Can you work these out from the model? Positions are in its coordinate system, mm. A direction names the side the tool comes from. Coordinates: 2 decimals unless noted, no trailing zeros. Order: outer loops, then holes, each group sorted by start corner. A loop starts at its lowest first (then second) coordinate and runs counter-clockwise, first axis right, second up. Notation, with made-up numbers: M 64.5,-38 L 72.5,-38 A25 cw 72.5,-22 Z; hole C 77.5,72.25 d2. An arc over 180 degrees is marked long. Answer as a JSON object with one key per item and string values.
from build123d import *

# Parameters (mm, degrees)
SKETCH1_R                           = 97.5
PLATE_DEPTH                         = 2
SKETCH2_W                           = 38
SKETCH2_H                           = 38
FIN_CLEARANCES_DEPTH                = 2
SKETCH3_W                           = 17.168411885
SKETCH3_H                           = 21
SERVO_CLEARANCE_DEPTH               = 2
SKETCH4_W                           = 4
SKETCH4_H                           = 21
SERVO_LIP_BOTTOM_DEPTH              = 8
SKETCH5_W                           = 10.5
SKETCH5_H                           = 5
SERVO_LIP_TOP_EXTRUSION_DEPTH       = 52
SKETCH6_W                           = 10.5
SKETCH6_H                           = 11.9
SERVO_LIP_TOP_DEPTH                 = 20.75
SKETCH7_W                           = 35
SKETCH7_H                           = 21
SERVO_CLEARANCE_FOR_INSERTION_DEPTH = 2
F_4_SERVO_LIP_EXTRUSIONS_COUNT      = 4
SKETCH8_W                           = 10.5
SKETCH8_H                           = 11.9
BOSS_EXTRUDE6_DEPTH                 = 20.75
SKETCH9_W                           = 10.5
SKETCH9_H                           = 11.9
BOSS_EXTRUDE7_DEPTH                 = 20.75
SKETCH10_W                          = 10.5
SKETCH10_H                          = 11.9
BOSS_EXTRUDE8_DEPTH                 = 20.75
SKETCH11_W                          = 5
SKETCH11_H                          = 55
EBOX_LID_SUPPORT_DEPTH              = 50
CUT_EXTRUDE4_DEPTH                  = 2
CLIP_CLEARANCES_COUNT               = 4
SKETCH13_W                          = 6
SKETCH13_H                          = 89.5
EBOX_BOTTOM_SUPPORT_DEPTH           = 20
SKETCH14_W                          = 22
SKETCH14_H                          = 5
SKETCH14_W_2                        = 3
SKETCH14_H_2                        = 8
CUT_EXTRUDE5_DEPTH                  = 10
CIRPATTERN1_COUNT                   = 4


with BuildPart() as part:
    # Sketch1 → Plate (new body)
    with BuildSketch(Plane(origin=(0, 0, 0), x_dir=(1, 0, 0), z_dir=(0, 1, 0))):
        with Locations(Location((0, 0, 0), (0, 0, 270))):
            Circle(SKETCH1_R)
    extrude(amount=PLATE_DEPTH)

    # Sketch2 → Fin Clearances (cut)
    with BuildSketch(Plane(origin=(0, 2, 0), x_dir=(1, 0, 0), z_dir=(0, 1, 0))):
        with Locations((69, 0)):
            Rectangle(SKETCH2_W, SKETCH2_H)
        with Locations((0, 69)):
            Rectangle(SKETCH2_W, SKETCH2_H)
        with Locations((0, -69)):
            Rectangle(SKETCH2_W, SKETCH2_H)
        with Locations((-69, 0)):
            Rectangle(SKETCH2_W, SKETCH2_H)
    extrude(amount=-FIN_CLEARANCES_DEPTH, mode=Mode.SUBTRACT)

    # Sketch3 → Servo Clearance (cut)
    with BuildSketch(Plane.XZ):
        with Locations((-27.584205943, -55.25)):
            Rectangle(SKETCH3_W, SKETCH3_H)
    servo_clearance = extrude(amount=-SERVO_CLEARANCE_DEPTH, mode=Mode.SUBTRACT)

    # Sketch4 → Servo Lip - Bottom (add)
    with BuildSketch(Plane.XZ):
        with Locations((-38.168411885, -55.25)):
            Rectangle(SKETCH4_W, SKETCH4_H)
    servo_lip_bottom = extrude(amount=SERVO_LIP_BOTTOM_DEPTH)

    # Sketch5 → Servo Lip - Top Extrusion (add)
    with BuildSketch(Plane(origin=(0, 2, 0), x_dir=(1, 0, 0), z_dir=(0, 1, 0))):
        with Locations((-41.418411885, 68.25)):
            Rectangle(SKETCH5_W, SKETCH5_H)
    servo_lip_top_extrusion = extrude(amount=SERVO_LIP_TOP_EXTRUSION_DEPTH)

    # Sketch6 → Servo Lip - Top (add)
    with BuildSketch(Plane.XY.offset(-65.75)):
        with Locations((-41.418411885, 48.05)):
            Rectangle(SKETCH6_W, SKETCH6_H)
    extrude(amount=SERVO_LIP_TOP_DEPTH)

    # Sketch7 → Servo Clearance for Insertion (cut)
    with BuildSketch(Plane.XZ):
        with Locations((-18.668411885, -55.25)):
            Rectangle(SKETCH7_W, SKETCH7_H)
    servo_clearance_for_insertion = extrude(amount=-SERVO_CLEARANCE_FOR_INSERTION_DEPTH, mode=Mode.SUBTRACT)

    # 4 Servo Lip Extrusions: Servo Clearance, Servo Lip - Bottom, Servo Lip - Top Extrusion, Servo Clearance for Insertion ×4 about axis
    f_4_servo_lip_extrusions_axis = Axis((0, 0, 0), (0, 1, 0))
    add([servo_clearance.rotate(f_4_servo_lip_extrusions_axis, i * 360 / F_4_SERVO_LIP_EXTRUSIONS_COUNT) for i in range(1, F_4_SERVO_LIP_EXTRUSIONS_COUNT)], mode=Mode.SUBTRACT)
    add([servo_lip_bottom.rotate(f_4_servo_lip_extrusions_axis, i * 360 / F_4_SERVO_LIP_EXTRUSIONS_COUNT) for i in range(1, F_4_SERVO_LIP_EXTRUSIONS_COUNT)])
    add([servo_lip_top_extrusion.rotate(f_4_servo_lip_extrusions_axis, i * 360 / F_4_SERVO_LIP_EXTRUSIONS_COUNT) for i in range(1, F_4_SERVO_LIP_EXTRUSIONS_COUNT)])
    add([servo_clearance_for_insertion.rotate(f_4_servo_lip_extrusions_axis, i * 360 / F_4_SERVO_LIP_EXTRUSIONS_COUNT) for i in range(1, F_4_SERVO_LIP_EXTRUSIONS_COUNT)], mode=Mode.SUBTRACT)

    # Sketch8 → Boss-Extrude6 (add)
    with BuildSketch(Plane(origin=(-65.75, 0, 0), x_dir=(0, 0, -1), z_dir=(1, 0, 0))):
        with Locations((-41.418411885, 48.05)):
            Rectangle(SKETCH8_W, SKETCH8_H)
    extrude(amount=BOSS_EXTRUDE6_DEPTH)

    # Sketch9 → Boss-Extrude7 (add)
    with BuildSketch(Plane(origin=(0, 0, 65.75), x_dir=(-1, 0, 0), z_dir=(0, 0, -1))):
        with Locations((-41.418411885, 48.05)):
            Rectangle(SKETCH9_W, SKETCH9_H)
    extrude(amount=BOSS_EXTRUDE7_DEPTH)

    # Sketch10 → Boss-Extrude8 (add)
    with BuildSketch(Plane.ZY.offset(-65.75)):
        with Locations((-41.418411885, 48.05)):
            Rectangle(SKETCH10_W, SKETCH10_H)
    extrude(amount=BOSS_EXTRUDE8_DEPTH)

    # Sketch11 → EBox Lid Support (add)
    with BuildSketch(Plane(origin=(0, 2, 0), x_dir=(1, 0, 0), z_dir=(0, 1, 0))):
        with Locations((-30.25, -1.627343475)):
            Rectangle(SKETCH11_W, SKETCH11_H)
    extrude(amount=EBOX_LID_SUPPORT_DEPTH)

    # Sketch12 → Cut-Extrude4 (cut)
    with BuildSketch(Plane.XZ):
        Polygon((-71.064231509, 63.993163697), (-63.993163697, 71.064231509), (-65.40737726, 72.478445072), (-72.478445072, 65.40737726), align=None)
    cut_extrude4 = extrude(amount=-CUT_EXTRUDE4_DEPTH, mode=Mode.SUBTRACT)

    # Clip Clearances: Cut-Extrude4 ×4 about axis
    clip_clearances_axis = Axis((0, 0, 0), (0, 1, 0))
    for i in range(1, CLIP_CLEARANCES_COUNT):
        add(cut_extrude4.rotate(clip_clearances_axis, i * 360 / CLIP_CLEARANCES_COUNT), mode=Mode.SUBTRACT)

    # Sketch13 → EBox Bottom Support (add)
    with BuildSketch(Plane(origin=(0, 2, 0), x_dir=(1, 0, 0), z_dir=(0, 1, 0))):
        with Locations((31, 0)):
            Rectangle(SKETCH13_W, SKETCH13_H)
    extrude(amount=EBOX_BOTTOM_SUPPORT_DEPTH)

    # Sketch14 → Cut-Extrude5 (cut)
    with BuildSketch(Plane.XZ):
        with Locations((51.168411885, 55.25)):
            Rectangle(SKETCH14_W, SKETCH14_H)
        with Locations((60.5, 38)):
            Rectangle(SKETCH14_W_2, SKETCH14_H_2)
    cut_extrude5 = extrude(amount=-CUT_EXTRUDE5_DEPTH, mode=Mode.SUBTRACT)

    # CirPattern1: Cut-Extrude5 ×4 about axis
    cirpattern1_axis = Axis((0, 0, 0), (0, 1, 0))
    for i in range(1, CIRPATTERN1_COUNT):
        add(cut_extrude5.rotate(cirpattern1_axis, i * 360 / CIRPATTERN1_COUNT), mode=Mode.SUBTRACT)


solid = part.part
Item 1: Please list where these lines run through material, in increasing order: line 1 (Z direction, x = 46, y = 43.5); line 2 (Z direction, x = -53, y = 47); line 3 (X direction, y = 30, z = -20.5).
Answers follow:
{"line 1": "z = -46.67 to -36.17, 45 to 70.75", "line 2": "z = 36.17 to 46.67", "line 3": "x = -32.75 to -27.75"}
Item 2: I want a section at B-B, the plane y = 32. Write out the boundary of the cut face in (x, z).
Answers follow:
{"outline": "M -70.75,36.17 L -65.75,36.17 L -65.75,46.67 L -70.75,46.67 Z; M -46.67,-70.75 L -36.17,-70.75 L -36.17,-65.75 L -46.67,-65.75 Z; M -32.75,-25.87 L -27.75,-25.87 L -27.75,29.13 L -32.75,29.13 Z; M 36.17,65.75 L 46.67,65.75 L 46.67,70.75 L 36.17,70.75 Z; M 65.75,-46.67 L 70.75,-46.67 L 70.75,-36.17 L 65.75,-36.17 Z"}
Item 3: I'm going to push flat-ended pins straight in: pin 1 (8 mm diameter, centred on y = -2, z = 56.5, fed in from -X); pin 2 (4.5 mm diameter, centred on x = -39, y = -4.5, fed in from -Z); pin 3 (4 mm diameter, centred on y = 19, z = 8.5, fed in from +X). Where does each tip first touch, or does it pass through?
Answers follow:
{"pin 1": "stops at x = -81.81", "pin 2": "stops at z = -65.75", "pin 3": "stops at x = 34"}
Item 4: I want a section at D-D, the plane x = -7.5. Write out the boundary of the cut face in (y, z).
Answers follow:
{"outline": "M 0,-97.21 L 2,-97.21 L 2,-88 L 0,-88 Z; M 0,-44.75 L 2,-44.75 L 2,50 L 0,50 Z; M 0,88 L 2,88 L 2,97.21 L 0,97.21 Z"}
Item 5: I want a section at C-C, the plane z = -29.5. Write out the boundary of the cut face in (x, y), plus the area to 3 significant figures.
Answers follow:
{"outline": "M -92.93,0 L 44.75,0 L 44.75,2 L 34,2 L 34,22 L 28,22 L 28,2 L -92.93,2 Z; M 65.75,0 L 92.93,0 L 92.93,2 L 65.75,2 Z", "area": "450 mm^2"}
Item 6: If we mould it in two halves opening along Z, with no side actions, what happens to faces 5 (the flat face through (67, 39, -46.668)), 6 (the flat face through (-67, 39, 46.668)), 7 (the flat face through (65.75, 22, -41)), 8 (the flat face through (36.168, -3, 55))? For each: pulls with the +Z half, pulls with the -Z half, needs draft (parallel to the pull), parting line crosses it, or undercut.
Answers follow:
{"face 5": "pulls with the -Z half", "face 6": "pulls with the +Z half", "face 7": "needs draft", "face 8": "undercut"}
Item 7: Which directions (+Z, -Z, +X, -X, +Y, -Y) give clear straight access to the entire face, cutting with the end or side of a thin tool? Please do faces 1 (the flat face through (-65.75, 22, 41)), 2 (the flat face through (67.58, 0.99, -67.48)), 3 (the cylindrical face through (-97.495, 0.986, -1.002)), 4 (the flat face through (70.75, 28, -41)).
Answers follow:
{"face 1": "+Z, -Z", "face 2": "+Y, -Y", "face 3": "-X, +Y, -Y", "face 4": "+Z, -Z, +X, +Y"}
Item 8: I want a section at A-A, the plane y = 15. Write out the boundary of the cut face in (x, z), plus the area to 3 significant figures.
Answers follow:
{"outline": "M -70.75,36.17 L -65.75,36.17 L -65.75,46.67 L -70.75,46.67 Z; M -46.67,-70.75 L -36.17,-70.75 L -36.17,-65.75 L -46.67,-65.75 Z; M -32.75,-25.87 L -27.75,-25.87 L -27.75,29.13 L -32.75,29.13 Z; M 28,-44.75 L 34,-44.75 L 34,44.75 L 28,44.75 Z; M 36.17,65.75 L 46.67,65.75 L 46.67,70.75 L 36.17,70.75 Z; M 65.75,-46.67 L 70.75,-46.67 L 70.75,-36.17 L 65.75,-36.17 Z", "area": "1,020 mm^2"}
